Study the drawing (mm; zero at the part's minimum x, y, z) and answer. Coordinates: 2 decimals unless noted, no trailing zeros. Order: outer loops, then holes, each group sorted by start corner. A loop starts at its lowest first (then second) coordinate and runs counter-clockwise, first axis right, second up.
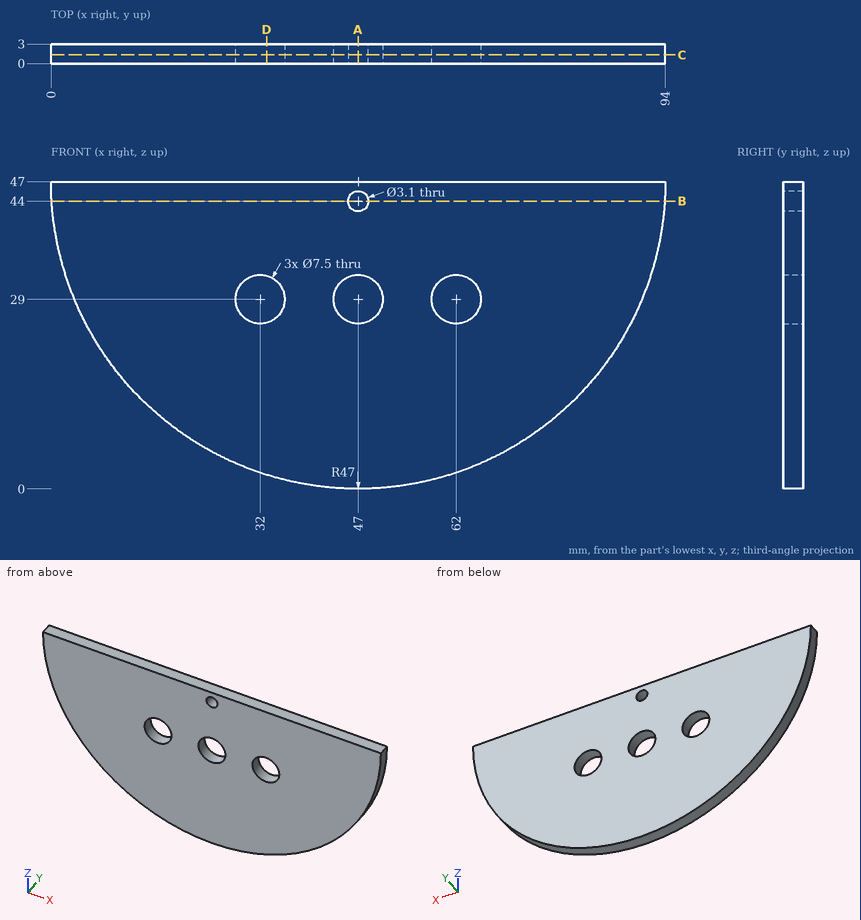
(1) Find section C-C on y = 1.35. Determine the outline of the cut face in (x, z), then the cut area to 3 significant figures.
(2) Find section B-B on z = 44. Determine the outline of the cut face in (x, y).
(3) Find section A-A on x = 47. Determine the outline of the cut face in (y, z), then the cut area to 3 significant figures.
(4) Find the intervals of material crossed by probe 1 along Z at (x, y) = (47, 1.55); probe 2 along X at (y, z) = (1.8, 29); probe 3 along Z at (x, y) = (62, 1.55), in increasing order.
(5) Find section D-D on x = 33. Determine the outline of the cut face in (y, z), then the cut area to 3 significant figures.
Resolved:
1. outline: (0, 47) arc R47 ccw to (94, 47) - close; hole circle Ø7.5 at (32, 29); hole circle Ø7.5 at (47, 29); hole circle Ø3.1 at (47, 44); hole circle Ø7.5 at (62, 29)
1. area: 3,330 mm2
2. outline: (0.1, 0) - (45.45, 0) - (45.45, 3) - (0.1, 3) - close; (48.55, 0) - (93.9, 0) - (93.9, 3) - (48.55, 3) - close
3. outline: (0, 0) - (3, 0) - (3, 25.25) - (0, 25.25) - close; (0, 32.75) - (3, 32.75) - (3, 42.45) - (0, 42.45) - close; (0, 45.55) - (3, 45.55) - (3, 47) - (0, 47) - close
3. area: 109 mm2
4. probe 1: z = 0 to 25.25, 32.75 to 42.45, 45.55 to 47
4. probe 2: x = 3.58 to 28.25, 35.75 to 43.25, 50.75 to 58.25, 65.75 to 90.42
4. probe 3: z = 2.46 to 25.25, 32.75 to 47
5. outline: (0, 2.13) - (3, 2.13) - (3, 25.39) - (0, 25.39) - close; (0, 32.61) - (3, 32.61) - (3, 47) - (0, 47) - close
5. area: 113 mm2
